The listing builds one solid part. Answer for the finished solid, in the listing's coordinates (mm). A direction names the side the tool comes from. Round coordinates to 2 decimals unless told otherwise and drop trailing zeros. Loops run counter-clockwise (first coordinate to the right, second up) from the corner with the lowest first, then second, coordinate; pieces in that order, holes last. Notation, with made-up numbers: M 13,2 L 45,2 A16 ccw 45,22 Z; hole C 33.5,34.5 d2. An arc over 180 degrees is marked long. Put each result on its own line as item: value. Start each with the question number.
(1) Determine the mould class of faces 1 (the face through (25.432, -0.282, 0.224)), 2 (the face through (0, -19, 24)), 3 (the face through (0, 30, 18)), 4 (the face through (6, -13, -16)) for opening direction Z: released by +Z, released by -Z, zero draft, split by the parting line, or undercut.
(2) Section C-C, the plane x = -6.5 is taken. Determine the outline of the cut face in (y, z), then the cut area to 3 significant figures.
(3) Straight lines are drawn through the part: line 1 (Z direction, x = 0, y = -22.5); line 2 (Z direction, x = -12.5, y = -25); line 3 (Z direction, x = 1.5, y = -23). For each, find the intervals that lie inside material, in ascending order.
(4) Flat-ended cylindrical pins translate along their axes: P1, Ø1.5, axis at x = -3, y = 19.5, coming from the -Z side; P2, Ø12, axis at x = 15, z = -11.5, coming from the +Y side; P3, Ø5, axis at y = -19, z = -5.5, coming from the -X side; P4, Ø4, axis at x = 20.5, z = 20.5, coming from the +Y side. Find the tip coordinate at first contact, or state that the pin passes through.
(5) Section A-A, the plane x = 0 is taken. Determine the outline of the cut face in (y, z).
(6) Which of the six approach directions +Z, -Z, +X, -X, +Y, -Y give full straight-line access (tool end or side, diameter ignored) to faces 5 (the face through (18, 15, 23)), 6 (the face through (23, 7, 20)), 7 (the face through (12, 13, 23))?
(7) Section D-D, the plane y = 21.5 is taken. Determine the outline of the cut face in (x, z).
(8) Section B-B, the plane y = -2.5 is taken. Determine the outline of the cut face in (x, z), then the cut area to 3 significant figures.
```python
from build123d import *

# Parameters (mm, degrees)
SALIENTE_EXTRUIR5_DEPTH  = 19
CORTAR_EXTRUIR8_DEPTH    = 16
SALIENTE_EXTRUIR8_DEPTH  = 3
REVOLUCI_N7_ANGLE        = 180
SALIENTE_EXTRUIR10_DEPTH = 15
CORTAR_EXTRUIR7_START    = 22
CORTAR_EXTRUIR7_DEPTH    = 2


with BuildPart() as part:
    # Croquis1 → Saliente-Extruir5 (new body, symmetric)
    with BuildSketch(Plane.XY):
        with BuildLine():
            Line((-27, 30), (-21.336320434, 30))
            ThreePointArc((-21.336320434, 30), (-19.399015955, 29.290600654), (-18.377926496, 27.497900903))
            Line((-18.377926496, 27.497900903), (-13.75, 0))
            ThreePointArc((-13.75, 0), (0, -13.75), (13.75, 0))
            Line((13.75, 0), (18.377926496, 27.497900903))
            ThreePointArc((18.377926496, 27.497900903), (19.399015955, 29.290600654), (21.336320434, 30))
            Line((21.336320434, 30), (27, 30))
            ThreePointArc((27, 30), (29.121320344, 29.121320344), (30, 27))
            Line((30, 27), (24, -30))
            Line((24, -30), (-24, -30))
            Line((-24, -30), (-30, 27))
            ThreePointArc((-30, 27), (-29.121320344, 29.121320344), (-27, 30))
        make_face()
    extrude(amount=SALIENTE_EXTRUIR5_DEPTH, both=True)

    # Croquis22 → Cortar-Extruir8 (cut, symmetric)
    with BuildSketch(Plane.XY):
        with BuildLine():
            Line((16, -30), (-16, -30))
            ThreePointArc((-16, -30), (-25.355108055, -0.70676981), (-27, 30))
            Line((-27, 30), (-18, 30))
            Line((-18, 30), (-13.75, 0))
            ThreePointArc((-13.75, 0), (0, -13.75), (13.75, 0))
            Line((13.75, 0), (18, 30))
            Line((18, 30), (27, 30))
            ThreePointArc((27, 30), (25.355108055, -0.70676981), (16, -30))
        make_face()
    extrude(amount=CORTAR_EXTRUIR8_DEPTH, both=True, mode=Mode.SUBTRACT)

    # Croquis8 → Saliente-Extruir8 (add)
    with BuildSketch(Plane.XY.offset(19)):
        Polygon((-21.336320434, 30), (21.336320434, 30), (21.336320434, -14), (0, -13.75), (-21.336320434, -14), align=None)
    extrude(amount=-SALIENTE_EXTRUIR8_DEPTH)

    # Croquis16 → Revolución7 (revolve)
    with BuildSketch(Plane(origin=(0, 0, 0), x_dir=(1, 0, 0), z_dir=(0, 1, 0))):
        Polygon((0, -22), (0, -24), (-25, -24), (-25, -19), (-23, -19), (-23, -22), align=None)
    revolve(axis=Axis((0, 0, 22), (0, 0, 1)), revolution_arc=REVOLUCI_N7_ANGLE)

    # Croquis18 → Saliente-Extruir10 (add)
    with BuildSketch(Plane(origin=(0, 0, 0), x_dir=(1, 0, 0), z_dir=(0, 1, 0))):
        Polygon((-25, -24), (25, -24), (25, -19), (23, -19), (23, -22), (-23, -22), (-23, -19), (-25, -19), align=None)
    extrude(amount=SALIENTE_EXTRUIR10_DEPTH)

    # Croquis19 → Cortar-Extruir7 (cut)
    with BuildSketch(Plane.XY.offset(CORTAR_EXTRUIR7_START)):
        with BuildLine():
            Line((-12, 10.5), (-12, 15))
            Line((-12, 15), (12, 15))
            Line((12, 15), (12, 10.5))
            ThreePointArc((12, 10.5), (0, -15.945218719), (-12, 10.5))
        make_face()
    extrude(amount=CORTAR_EXTRUIR7_DEPTH, mode=Mode.SUBTRACT)


solid = part.part
```
Recorded:
1. face 1: undercut
1. face 2: released by +Z
1. face 3: zero draft
1. face 4: undercut
2. outline: M -30,-19 L -12.12,-19 L -12.12,-16 L -30,-16 Z; M -30,16 L 30,16 L 30,19 L -22.06,19 L -22.06,22 L -14.56,22 L -14.56,24 L -24.14,24 L -24.14,19 L -30,19 Z
2. area: 259 mm²
3. line 1: z = -19 to -16, 16 to 19, 22 to 24
3. line 2: z = -19 to -16, 16 to 19
3. line 3: z = -19 to -16, 16 to 24
4. P1: stops at z = 16
4. P2: stops at y = 28.84
4. P3: stops at x = -25.42
4. P4: stops at y = 30
5. outline: M -30,-19 L -13.75,-19 L -13.75,-16 L -30,-16 Z; M -30,16 L 30,16 L 30,19 L -23,19 L -23,22 L -15.95,22 L -15.95,24 L -25,24 L -25,19 L -30,19 Z
6. face 5: +Z, +X, -X, +Y
6. face 6: +Y
6. face 7: +Z, +Y
7. outline: M -29.42,-19 L -17.37,-19 L -17.37,-16 L -27.33,-16 L -27.33,16 L 27.33,16 L 27.33,-16 L 17.37,-16 L 17.37,-19 L 29.42,-19 L 29.42,19 L -29.42,19 Z
8. outline: M -26.89,-19 L -13.52,-19 L -13.52,-16 L -25.01,-16 L -25.01,16 L 25.01,16 L 25.01,-16 L 13.52,-16 L 13.52,-19 L 26.89,-19 L 26.89,19 L 24.87,19 L 24.87,24 L 15.75,24 L 15.75,22 L 22.86,22 L 22.86,19 L -22.86,19 L -22.86,22 L -15.75,22 L -15.75,24 L -24.87,24 L -24.87,19 L -26.89,19 Z
8. area: 411 mm²
